For this review, take the finished solid that the model builds, in its own axes (mm). A direction names the side the tool comes from. Round coordinates to 2 decimals unless told otherwise and drop trailing zeros. Loops run counter-clockwise (first coordinate to the right, second up) from the corner with the lowest first, then second, coordinate; pieces in that order, holes last.
1. To check wall thickness, follow line 1 along Y through (x, z) = (2.75, 1.4); line 2 along X through (y, z) = (-6.5, 3); line 3 along Y through (x, z) = (4.5, 2.5). State the ranges of each line that lie inside material, in increasing order.
2. Consider section C-C on y = -2.75. State the section outline as (x, z) points (3 decimals).
3. Draft analysis for pull direction Y (two halves, no side actions). For faces 1 (the cylindrical face through (6.514, 8.925, 2.114)), 2 (the flat face through (0, -12.5, 1)), 3 (the flat face through (0, -4, 2)), 4 (the cylindrical face through (-3.075, -10.714, 1.014)), state which applies: released by +Y, released by -Y, zero draft, split by the parting line, or undercut.
4. Clearance check with flat-ended pins moving along their axes: pin 1 Ø1 at (x, y) = (4.5, 10.5) entering from +Z; pin 2 Ø2 at (x, z) = (3, 4.5) entering from +Y; pin 3 Ø0.6 at (x, z) = (5, 0.5) entering from +Y; pin 4 Ø4 at (x, y) = (2.75, -9.25) entering from +Z. State where each tip first meets the part, or that it passes through.
5. Consider section B-B on z = 1.25. State the section outline as (x, y) points, then the cut area to 3 significant figures.
6. Consider section A-A on x = -2.75. State the section outline as (y, z) points, then the cut area to 3 significant figures.
7. Tool access review of faces 5 (the flat face through (5, 0.5, 5)), 6 (the flat face through (4, 11, 2)), 7 (the flat face through (-7, 2.5, 4)), 8 (the flat face through (0, 3.5, 1)), 9 (the flat face through (6, 2.5, 4)): name each direction out of +Z, -Z, +X, -X, +Y, -Y from which nothing blocks a thin tool from reaching the whole face with its end or side.
8. Consider section D-D on y = 10.25. State the section outline as (x, z) points.
from build123d import *

# Parameters (mm, degrees)
SKETCH_1_W          = 15
SKETCH_1_H          = 25
EXTRUDE_1_DEPTH     = 7
CUT_EXTRUDE_1_DEPTH = 5
SKETCH_3_W          = 2
SKETCH_3_H          = 10
CUT_EXTRUDE_2_DEPTH = 13
SKETCH_4_W          = 2
SKETCH_4_H          = 3
CUT_EXTRUDE_3_DEPTH = 20.345542122
SKETCH_5_W          = 7
SKETCH_5_H          = 6
CUT_EXTRUDE_4_DEPTH = 13
SKETCH_6_R          = 1.5
EXTRUDE_2_DEPTH     = 2
EXTRUDE_START       = 2
SKETCH_7_R          = 1.5
EXTRUDE_3_DEPTH     = 2
CUT_EXTRUDE_5_DEPTH = 21.742468513
SKETCH_9_R          = 1.5
CUT_EXTRUDE_6_DEPTH = 16.411035007


with BuildPart() as part:
    # Эскиз1 → Бобышка-Вытянуть1 (new body)
    with BuildSketch(Plane.XY):
        Rectangle(SKETCH_1_W, SKETCH_1_H)
    extrude(amount=EXTRUDE_1_DEPTH)

    # Эскиз2 → Вырез-Вытянуть1 (cut)
    with BuildSketch(Plane.XY.offset(7)):
        Polygon((-3.5, 0.5), (-5.5, 0.5), (-5.5, -12.5), (5.5, -12.5), (5.5, 0.5), (3.5, 0.5), (3.5, 12.5), (-3.5, 12.5), align=None)
    extrude(amount=-CUT_EXTRUDE_1_DEPTH, mode=Mode.SUBTRACT)

    # Эскиз3 → Вырез-Вытянуть2 (cut)
    with BuildSketch(Plane.XY.offset(7)):
        with Locations((-6.5, 7.5)):
            Rectangle(SKETCH_3_W, SKETCH_3_H)
        with Locations((6.5, 7.5)):
            Rectangle(SKETCH_3_W, SKETCH_3_H)
    extrude(amount=-CUT_EXTRUDE_2_DEPTH, mode=Mode.SUBTRACT)

    # Эскиз4 → Вырез-Вытянуть3 (cut, through all)
    with BuildSketch(Plane.ZY.offset(5.5)):
        with Locations((6, 11)):
            Rectangle(SKETCH_4_W, SKETCH_4_H)
        with Locations((1, 11)):
            Rectangle(SKETCH_4_W, SKETCH_4_H)
    extrude(amount=-CUT_EXTRUDE_3_DEPTH, mode=Mode.SUBTRACT)

    # Эскиз5 → Вырез-Вытянуть4 (cut)
    with BuildSketch(Plane.XY.offset(2)):
        with Locations((0, 6.5)):
            Rectangle(SKETCH_5_W, SKETCH_5_H)
    extrude(amount=-CUT_EXTRUDE_4_DEPTH, mode=Mode.SUBTRACT)

    # Эскиз6 → Бобышка-Вытянуть2 (add)
    with BuildSketch(Plane.ZY.offset(5.5)):
        with Locations(Location((3.5, 9.5, 0), (0, 0, 180))):
            Circle(SKETCH_6_R)
    extrude(amount=EXTRUDE_2_DEPTH)

    # Эскиз7 → Бобышка-Вытянуть3 (add)
    with BuildSketch(Plane(origin=(5.5, 0, 0), x_dir=(0, 0, -1), z_dir=(1, 0, 0)).offset(EXTRUDE_START)):
        with Locations((-3.5, 9.5)):
            Circle(SKETCH_7_R)
    extrude(amount=-EXTRUDE_3_DEPTH)

    # Эскиз8 → Вырез-Вытянуть5 (cut, through all)
    with BuildSketch(Plane.ZY.offset(7.5)):
        Polygon((7, 0.5), (3.5, -12.5), (7, -12.5), align=None)
    extrude(amount=-CUT_EXTRUDE_5_DEPTH, mode=Mode.SUBTRACT)

    # Эскиз9 → Вырез-Вытянуть6 (cut, through all)
    with BuildSketch(Plane.XY.offset(2)):
        with Locations((-2.75, -2.75)):
            Circle(SKETCH_9_R)
        with Locations((2.75, -2.75)):
            Circle(SKETCH_9_R)
        with Locations((-2.75, -9.25)):
            Circle(SKETCH_9_R)
        with Locations((2.75, -9.25)):
            Circle(SKETCH_9_R)
    extrude(amount=-CUT_EXTRUDE_6_DEPTH, mode=Mode.SUBTRACT)


solid = part.part
Resolved:
1. line 1: y = -12.5 to -10.75, -7.75 to -4.25, -1.25 to 3.5
1. line 2: x = -7.5 to -5.5, 5.5 to 7.5
1. line 3: y = 0.5 to 12.5
2. outline: (-7.5, 0) - (-4.25, 0) - (-4.25, 2) - (-5.5, 2) - (-5.5, 6.125) - (-7.5, 6.125) - close; (-1.25, 0) - (1.25, 0) - (1.25, 2) - (-1.25, 2) - close; (4.25, 0) - (7.5, 0) - (7.5, 6.125) - (5.5, 6.125) - (5.5, 2) - (4.25, 2) - close
3. face 1: undercut
3. face 2: released by -Y
3. face 3: zero draft
3. face 4: undercut
4. pin 1: stops at z = 5
4. pin 2: stops at y = 12.5
4. pin 3: stops at y = 9.5
4. pin 4: stops at z = 2
5. outline: (-7.5, -12.5) - (7.5, -12.5) - (7.5, 2.5) - (5.5, 2.5) - (5.5, 9.5) - (3.5, 9.5) - (3.5, 3.5) - (-3.5, 3.5) - (-3.5, 9.5) - (-5.5, 9.5) - (-5.5, 2.5) - (-7.5, 2.5) - close; hole circle Ø3 at (-2.75, -9.25); hole circle Ø3 at (-2.75, -2.75); hole circle Ø3 at (2.75, -9.25); hole circle Ø3 at (2.75, -2.75)
5. area: 232 mm2
6. outline: (-12.5, 0) - (-10.75, 0) - (-10.75, 2) - (-12.5, 2) - close; (-7.75, 0) - (-4.25, 0) - (-4.25, 2) - (-7.75, 2) - close; (-1.25, 0) - (3.5, 0) - (3.5, 2) - (-1.25, 2) - close
6. area: 20.0 mm2
7. face 5: +Z, -Y
7. face 6: -Z, +X, -X, +Y
7. face 7: +Z, -Z, -X
7. face 8: +Z, -Z, +Y
7. face 9: +Z, -Z, +X
8. outline: (-7.5, 2.2) - (-5.5, 2.2) - (-5.5, 2) - (-3.5, 2) - (-3.5, 5) - (-5.5, 5) - (-5.5, 4.8) - (-7.5, 4.8) - close; (3.5, 2) - (5.5, 2) - (5.5, 2.2) - (7.5, 2.2) - (7.5, 4.8) - (5.5, 4.8) - (5.5, 5) - (3.5, 5) - close
